```python
from build123d import *

# Parameters (mm, degrees)
SKETCH1_W           = 9.23810595
SKETCH1_H           = 28.3
SKETCH1_W_2         = 22.995276356
SKETCH1_H_2         = 6.447183695
BOSS_EXTRUDE1_DEPTH = 5


with BuildPart() as part:
    # Sketch1 → Boss-Extrude1 (new body)
    with BuildSketch(Plane(origin=(0, 0, 0), x_dir=(1, 0, 0), z_dir=(0, 1, 0))):
        Polygon((-84.64385089, 36.855414935), (-89.512192258, 32.332884436), (-89.512192258, -81.365540516), (10.487807742, -81.365540516), (10.487807742, 32.332884436), (-10.408953914, 52.490004223), (-69.009261602, 52.490004223), align=None)
        with Locations((-65.864023501, 2.411444329)):
            Rectangle(SKETCH1_W, SKETCH1_H, mode=Mode.SUBTRACT)
        with Locations((-39.648008145, 28.020058308)):
            Rectangle(SKETCH1_W_2, SKETCH1_H_2, mode=Mode.SUBTRACT)
        with Locations((-13.554192015, 2.411444329)):
            Rectangle(SKETCH1_W, SKETCH1_H, mode=Mode.SUBTRACT)
    extrude(amount=BOSS_EXTRUDE1_DEPTH)


solid = part.part
```
The model under review builds one solid part; all positions refer to its coordinate system, in mm. A direction names the side the tool comes from. Round coordinates to 2 decimals unless told otherwise and drop trailing zeros. Loops run counter-clockwise (first coordinate to the right, second up) from the corner with the lowest first, then second, coordinate; pieces in that order, holes last. Notation, with made-up numbers: (4.25, -26.75) -> (17.25, -26.75) arc R29 cw to (17.25, -5.75) -> close; hole circle Ø9 at (30.25, 45.25). An arc over 180 degrees is marked (long way). Answer in a Markdown table with one row per item.
1) For pin 1 Ø3 at (x, y) = (-79, 4.5) entering from -Z, flat-tipped, find the tip position at first contact; note if it passes through.
Taken from the geometry:
| item | result |
|---|---|
| pin 1 | stops at z = -44 |
2) Wall thickness on line 1 along X through (y, z) = (0.5, -13.5); line 2 along Z through (x, y) = (-44, 1.6); line 3 along X through (y, z) = (4.15, -27): over which ranges is each line inside the solid? List them lowest first.
Taken from the geometry:
| item | result |
|---|---|
| line 1 | x = -89.51 to -70.48, -61.24 to -18.17, -8.94 to 10.49 |
| line 2 | z = -52.49 to -31.24, -24.8 to 81.37 |
| line 3 | x = -89.51 to -51.15, -28.15 to 10.49 |
3) Consider section B-B, the plane x = -37. Write out the cut boundary in (y, z), plus the area to 3 significant figures.
Taken from the geometry:
| item | result |
|---|---|
| outline | (0, -52.49) -> (5, -52.49) -> (5, -31.24) -> (0, -31.24) -> close; (0, -24.8) -> (5, -24.8) -> (5, 81.37) -> (0, 81.37) -> close |
| area | 637 mm² |
4) Draft analysis for pull direction X (two halves, no side actions). For faces 1 (the flat face through (-40, 2, 81.366)), 2 (the flat face through (-61.245, 2, -2)), 3 (the flat face through (-87.04, 2.46, -34.63)), 4 (the flat face through (10.488, 2, 25)), state which applies: pulls with the +X half, pulls with the -X half, needs draft (parallel to the pull), parting line crosses it, or undercut.
Taken from the geometry:
| item | result |
|---|---|
| face 1 | needs draft |
| face 2 | undercut |
| face 3 | pulls with the -X half |
| face 4 | pulls with the +X half |
5) Consider section D-D, the plane z = -4. Write out the cut boundary in (x, y).
Taken from the geometry:
| item | result |
|---|---|
| outline | (-89.51, 0) -> (-70.48, 0) -> (-70.48, 5) -> (-89.51, 5) -> close; (-61.24, 0) -> (-18.17, 0) -> (-18.17, 5) -> (-61.24, 5) -> close; (-8.94, 0) -> (10.49, 0) -> (10.49, 5) -> (-8.94, 5) -> close |
6) Consider section C-C, the plane y = 3.6. Write out the cut boundary in (x, z).
Taken from the geometry:
| item | result |
|---|---|
| outline | (-89.51, -32.33) -> (-84.64, -36.86) -> (-69.01, -52.49) -> (-10.41, -52.49) -> (10.49, -32.33) -> (10.49, 81.37) -> (-89.51, 81.37) -> close; hole (-70.48, -16.56) -> (-61.24, -16.56) -> (-61.24, 11.74) -> (-70.48, 11.74) -> close; hole (-51.15, -31.24) -> (-28.15, -31.24) -> (-28.15, -24.8) -> (-51.15, -24.8) -> close; hole (-18.17, -16.56) -> (-8.94, -16.56) -> (-8.94, 11.74) -> (-18.17, 11.74) -> close |
7) Tool access review of faces 5 (the flat face through (-28.15, 2, -28)), 6 (the flat face through (-40, 5, 14)): name each direction out of +Z, -Z, +X, -X, +Y, -Y from which nothing blocks a thin tool from reaching the whole face with its end or side.
Taken from the geometry:
| item | result |
|---|---|
| face 5 | +Y, -Y |
| face 6 | +Z, -Z, +X, -X, +Y |
8) Consider section A-A, the plane z = -28.5. Write out the cut boundary in (x, y).
Taken from the geometry:
| item | result |
|---|---|
| outline | (-89.51, 0) -> (-51.15, 0) -> (-51.15, 5) -> (-89.51, 5) -> close; (-28.15, 0) -> (10.49, 0) -> (10.49, 5) -> (-28.15, 5) -> close |
